from build123d import *

# Parameters (mm, degrees)
SKETCH1_R              = 6.35
BOSS_EXTRUDE1_DEPTH    = 50.8
SKETCH1_R_2            = 6.349999999999999
BOSS_EXTRUDE1_2_DEPTH  = 50.8
SKETCH1_R_3            = 6.350000000000002
BOSS_EXTRUDE1_3_DEPTH  = 50.8
BOSS_EXTRUDE1_4_DEPTH  = 50.8
BOSS_EXTRUDE1_5_DEPTH  = 50.8
BOSS_EXTRUDE1_6_DEPTH  = 50.8
BOSS_EXTRUDE1_7_DEPTH  = 50.8
SKETCH1_R_4            = 6.350000000000003
BOSS_EXTRUDE1_8_DEPTH  = 50.8
BOSS_EXTRUDE1_9_DEPTH  = 50.8
SKETCH1_R_5            = 6.3500000000000005
BOSS_EXTRUDE1_10_DEPTH = 50.8
BOSS_EXTRUDE2_DEPTH    = 1.27
BOSS_EXTRUDE3_DEPTH    = 0.0254


with BuildPart() as part:
    # Sketch1 → Boss-Extrude1 (new body)
    with BuildSketch(Plane(origin=(0, 0, 0), x_dir=(1, 0, 0), z_dir=(0, 1, 0))):
        with Locations(Location((0, 0, 0), (0, 0, 270))):
            Circle(SKETCH1_R)
    extrude(amount=BOSS_EXTRUDE1_DEPTH)



with BuildPart() as body_2:
    # Sketch1 → Boss-Extrude1 2 (new body)
    with BuildSketch(Plane(origin=(0, 0, 0), x_dir=(1, 0, 0), z_dir=(0, 1, 0))):
        with Locations(Location((12.954, 0, 0), (0, 0, 270))):
            Circle(SKETCH1_R_2)
    extrude(amount=BOSS_EXTRUDE1_2_DEPTH)


with BuildPart() as body_3:
    # Sketch1 → Boss-Extrude1 3 (new body)
    with BuildSketch(Plane(origin=(0, 0, 0), x_dir=(1, 0, 0), z_dir=(0, 1, 0))):
        with Locations(Location((25.908, 0, 0), (0, 0, 270))):
            Circle(SKETCH1_R_3)
    extrude(amount=BOSS_EXTRUDE1_3_DEPTH)


with BuildPart() as body_4:
    # Sketch1 → Boss-Extrude1 4 (new body)
    with BuildSketch(Plane(origin=(0, 0, 0), x_dir=(1, 0, 0), z_dir=(0, 1, 0))):
        with Locations(Location((38.862, 0, 0), (0, 0, 270))):
            Circle(SKETCH1_R_3)
    extrude(amount=BOSS_EXTRUDE1_4_DEPTH)


with BuildPart() as body_5:
    # Sketch1 → Boss-Extrude1 5 (new body)
    with BuildSketch(Plane(origin=(0, 0, 0), x_dir=(1, 0, 0), z_dir=(0, 1, 0))):
        with Locations(Location((51.816, 0, 0), (0, 0, 270))):
            Circle(SKETCH1_R_3)
    extrude(amount=BOSS_EXTRUDE1_5_DEPTH)


with BuildPart() as body_6:
    # Sketch1 → Boss-Extrude1 6 (new body)
    with BuildSketch(Plane(origin=(0, 0, 0), x_dir=(1, 0, 0), z_dir=(0, 1, 0))):
        with Locations(Location((12.954000000000136, -12.954, 0), (0, 0, 270))):
            Circle(SKETCH1_R)
    extrude(amount=BOSS_EXTRUDE1_6_DEPTH)


with BuildPart() as body_7:
    # Sketch1 → Boss-Extrude1 7 (new body)
    with BuildSketch(Plane(origin=(0, 0, 0), x_dir=(1, 0, 0), z_dir=(0, 1, 0))):
        with Locations(Location((25.908000000000136, -12.954, 0), (0, 0, 270))):
            Circle(SKETCH1_R)
    extrude(amount=BOSS_EXTRUDE1_7_DEPTH)


with BuildPart() as body_8:
    # Sketch1 → Boss-Extrude1 8 (new body)
    with BuildSketch(Plane(origin=(0, 0, 0), x_dir=(1, 0, 0), z_dir=(0, 1, 0))):
        with Locations(Location((38.86200000000014, -12.954, 0), (0, 0, 270))):
            Circle(SKETCH1_R_4)
    extrude(amount=BOSS_EXTRUDE1_8_DEPTH)


with BuildPart() as body_9:
    # Sketch1 → Boss-Extrude1 9 (new body)
    with BuildSketch(Plane(origin=(0, 0, 0), x_dir=(1, 0, 0), z_dir=(0, 1, 0))):
        with Locations(Location((51.81600000000014, -12.954, 0), (0, 0, 270))):
            Circle(SKETCH1_R_4)
    extrude(amount=BOSS_EXTRUDE1_9_DEPTH)


with BuildPart() as body_10:
    # Sketch1 → Boss-Extrude1 10 (new body)
    with BuildSketch(Plane(origin=(0, 0, 0), x_dir=(1, 0, 0), z_dir=(0, 1, 0))):
        with Locations(Location((1.3569e-13, -12.954, 0), (0, 0, 270))):
            Circle(SKETCH1_R_5)
    extrude(amount=BOSS_EXTRUDE1_10_DEPTH)


with BuildPart() as part_1:
    add(part.part)

    add(body_2.part)  # Boss-Extrude2 merges body 2

    add(body_3.part)  # Boss-Extrude2 merges body 3

    add(body_4.part)  # Boss-Extrude2 merges body 4

    add(body_5.part)  # Boss-Extrude2 merges body 5

    add(body_6.part)  # Boss-Extrude2 merges body 6

    add(body_7.part)  # Boss-Extrude2 merges body 7

    add(body_8.part)  # Boss-Extrude2 merges body 8

    add(body_9.part)  # Boss-Extrude2 merges body 9

    add(body_10.part)  # Boss-Extrude2 merges body 10
    # Sketch4 → Boss-Extrude2 (add)
    with BuildSketch(Plane(origin=(0, 50.8, 0), x_dir=(1, 0, 0), z_dir=(0, 1, 0))):
        with BuildLine():
            Line((1.3569e-13, -6.604), (0, -6.35))
            ThreePointArc((0, -6.35), (-4.490128060534576, 4.490128060534577), (6.35, 0))
            Line((6.35, 0), (6.603999999999998, 0))
            ThreePointArc((6.603999999999998, 0), (12.954, 6.350000000000001), (19.304000000000002, 0))
            Line((19.304000000000002, 0), (19.558, 0))
            ThreePointArc((19.558, 0), (25.908, 6.350000000000001), (32.258, 0))
            Line((32.258, 0), (32.512, 0))
            ThreePointArc((32.512, 0), (38.862, 6.350000000000001), (45.212, 0))
            Line((45.212, 0), (45.466, 0))
            ThreePointArc((45.466, 0), (56.30612806053458, 4.490128060534578), (51.816, -6.350000000000002))
            Line((51.816, -6.350000000000002), (51.81600000000014, -6.603999999999998))
            ThreePointArc((51.81600000000014, -6.603999999999998), (56.30612806053472, -17.44412806053458), (45.466000000000136, -12.954))
            Line((45.466000000000136, -12.954), (45.21200000000014, -12.954))
            ThreePointArc((45.21200000000014, -12.954), (38.86200000000014, -19.304000000000002), (32.512000000000135, -12.954))
            Line((32.512000000000135, -12.954), (32.25800000000013, -12.954))
            ThreePointArc((32.25800000000013, -12.954), (25.908000000000136, -19.304), (19.55800000000014, -12.954))
            Line((19.55800000000014, -12.954), (19.304000000000133, -12.954))
            ThreePointArc((19.304000000000133, -12.954), (12.954000000000134, -19.304), (6.604000000000137, -12.954))
            Line((6.604000000000137, -12.954), (6.350000000000135, -12.954))
            ThreePointArc((6.350000000000135, -12.954), (-4.490128060534443, -17.444128060534577), (1.3569e-13, -6.604))
        make_face()
    boss_extrude2 = extrude(amount=BOSS_EXTRUDE2_DEPTH)

    # Mirror1: Boss-Extrude2 across plane
    add(boss_extrude2.mirror(Plane.ZX.offset(25.4)))

    # Sketch5 → Boss-Extrude3 (add)
    with BuildSketch(Plane(origin=(0, 52.07, 0), x_dir=(1, 0, 0), z_dir=(0, 1, 0))):
        Polygon((51.81599999999998, 6.350000000000001), (-2.602e-14, 6.349999999999999), (-6.35, -4.434e-14), (-6.349999999999865, -12.954000000000045), (2.5457e-13, -19.304000000000002), (51.81600000000021, -19.304000000000002), (58.16600000000014, -12.95399999999983), (58.166000000000004, 0), align=None)
    boss_extrude3 = extrude(amount=BOSS_EXTRUDE3_DEPTH)

    # Mirror2: Boss-Extrude3 across plane
    add(boss_extrude3.mirror(Plane.ZX.offset(25.4)))


solid = part_1.part
Part model, mm, in its own coordinate system. A direction names the side the tool comes from. Coordinates: 2 decimals unless noted, no trailing zeros. Use a Markdown table: item, result. Add a question column.
Q1. Which spindle directions (+Z, -Z, +X, -X, +Y, -Y) get a long thin tool onto all of the face, cutting with end or side? Do faces 1 (the flat face through (25, 52.095, 6)), 2 (the cylindrical face through (28.27, 25.03, 18.85)). Say none if no direction does.
Q2. Pin check, flat tips, straight feed: P1, Ø1.5, axis at x = 33.5, y = 35, coming from the +Z side; P2, Ø4, axis at x = 18.5, y = 18.5, coming from the +Z side; P3, Ø1, axis at x = 47.5, y = 20, coming from the -Z side. Stop position of each tip, or through.
Q3. Probe L1, parallel to X at y = 8, z = 13; L2, parallel to X at y = 11, z = 12.5; L3, parallel to Y at x = 7, z = 7. List the from-to ranges inside material, lowest first.
Q4. Cut at A-A (y = 45.5). Give the number of separate pieces and of enclosed holes in the cut face, and give its area (3 significant figures).
Q5. Mould opens along X. For faces 3 (the flat face through (30, 50.8, 6)), 4 (the flat face through (55, 52.07, 17)) say: +X half, -X half, draft (parallel to the pull), parting line (faces both ways), or undercut.
Worked out:
| question | item | result |
|---|---|---|
| 1 | face 1 | +Z, -Z, +X, -X, +Y |
| 1 | face 2 | none |
| 2 | P1 | stops at z = 17.32 |
| 2 | P2 | stops at z = 18.22 |
| 2 | P3 | stops at z = -5.08 |
| 3 | L1 | x = -6.35 to 6.35, 6.6 to 19.3, 19.56 to 32.26, 32.51 to 45.21, 45.47 to 58.17 |
| 3 | L2 | x = -6.33 to 6.33, 6.62 to 19.29, 19.57 to 32.24, 32.53 to 45.2, 45.48 to 58.15 |
| 3 | L3 | y = -1.3 to 0, 50.8 to 52.1 |
| 4 | separate pieces | 10 |
| 4 | enclosed holes | 0 |
| 4 | area | 1,270 mm2 |
| 5 | face 3 | undercut |
| 5 | face 4 | draft |
